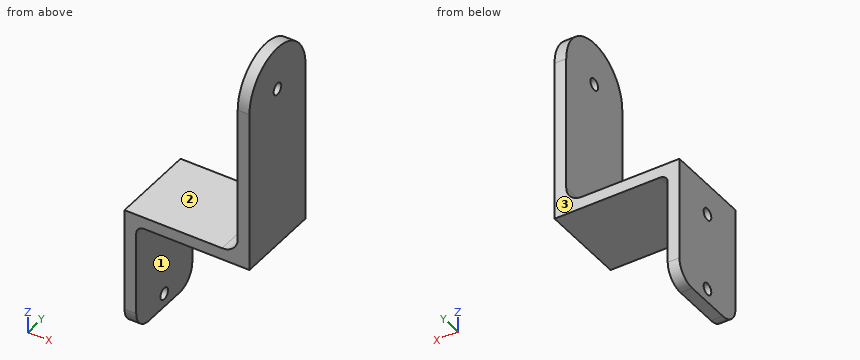
Autodesk Inventor part; units mm, degrees
ref_plane "YZ Plane" through (0, 0, 0) normal (1, 0, 0) x (0, 1, 0)
ref_plane "XZ Plane" through (0, 0, 0) normal (0, 1, 0) x (-1, 0, 0)
ref_plane "XY Plane" through (0, 0, 0) normal (0, 0, 1) x (1, 0, 0)
sketch "Sketch1" plane through (0, 0, 0) normal (1, 0, 0) x (0, 1, 0)
  circle A0 centre (0, 0) radius 1.5
  circle A1 centre (0, -20) radius 1.5
  line L0 (0, 0) -> (12, 0)
  line L1 (12, 0) -> (12, -20)
  line L2 (0, 0) -> (-12, 0)
  line L3 (-12, 0) -> (-12, -20)
  arc A2 (0, -16.5) -> (0, -23.5) centre (0, -20) ccw
  line L4 (12, -20) -> (12, -23.5)
  line L5 (12, -23.5) -> (-12, -23.5)
  line L6 (-12, -23.5) -> (-12, -20)
  line L7 (0, 0) -> (0, -1.5)
  line L8 (0, -16.5) -> (0, -20)
  line L9 (12, 0) -> (12, 5)
  line L10 (12, 5) -> (-12, 5)
  line L11 (-12, 5) -> (-12, 0)
  dimension "d0" = 3
  dimension "d1" = 20
  dimension "d2" = 3
  dimension "d3" = 12
  dimension "d4" = 12
  dimension "d5" = 7
  dimension "d6" = 5
extrude "Extrusion1" add sketch "Sketch1" along normal blind 3 contours A0 L0 L1 L4 L5 L6 L3 L2 | A0 L2 L11 L10 L9 L0
sketch "Sketch2" plane through (0, 0, 0) normal (-1, 0, 0) x (0, 0, 1)
  line L0 (-23.5, 12) -> (5, 12)
  line L1 (-23.5, -12) -> (-23.5, 12)
  line L2 (5, -12) -> (-23.5, -12)
  line L3 (5, 12) -> (5, -12)
  circle A0 centre (-20, 0) radius 1.5
  circle A1 centre (0, 0) radius 1.5
  line L4 (5, 12) -> (5, -12)
  line L5 (5, -12) -> (8, -12)
  line L6 (8, -12) -> (8, 12)
  line L7 (-23.5, 12) -> (5, 12)
  line L8 (8, 12) -> (5, 12)
  dimension "d9" = 3
extrude "Extrusion2" add sketch "Sketch2" against normal blind 32 contours L8 L6 L5 L3
sketch "Sketch3" plane through (0, -12, 8) normal (0, 0, 1) x (1, 0, 0)
  line L0 (0, 0) -> (0, 24)
  line L1 (0, 0) -> (32, 0)
  line L2 (32, 24) -> (32, 0)
  line L3 (0, 24) -> (32, 24)
  line L4 (32, 24) -> (32, 0)
  line L5 (32, 0) -> (29, 0)
  line L6 (0, 0) -> (32, 0)
  line L7 (29, 0) -> (29, 24)
  line L8 (0, 24) -> (32, 24)
  point P0 (0, 12)
  dimension "d12" = 3
extrude "Extrusion3" add sketch "Sketch3" along normal blind 50 contours L7 L3 L2 L1
sketch "Sketch4" plane through (32, 0, 0) normal (1, 0, 0) x (0, 0, -1)
  line L0 (-5, -12) -> (-5, 12)
  line L1 (-5, 12) -> (-58, 12)
  line L2 (-58, -12) -> (-58, 12)
  line L3 (-5, -12) -> (-58, -12)
  line L4 (23.5, 12) -> (-5, 12)
  line L5 (-5, 12) -> (-5, 0)
  line L6 (-5, -12) -> (-5, 12)
  line L7 (-5, 0) -> (-46.61, 0)
  circle A0 centre (-46.61, 0) radius 1.5
  point P0 (0, 0)
  dimension "d15" = 12
  dimension "d16" = 41.61
  dimension "d17" = 3
extrude "Extrusion4" cut sketch "Sketch4" against normal blind 50 contours A0
fillet "Fillet1" radius 2 1 edges at (3, 0, 5)
fillet "Fillet2" radius 4 1 edges at (29, 0, 8)
sketch "Sketch5" plane through (32, 0, 0) normal (1, 0, 0) x (0, 0, -1)
  circle A0 centre (-46.61, 0) radius 1.5
  line L0 (-5, -12) -> (-5, 12)
  line L1 (-5, 12) -> (-58, 12)
  line L2 (-58, -12) -> (-58, 12)
  line L3 (-5, -12) -> (-58, -12)
  circle A1 centre (-46.61, 0) radius 1.5
  circle A2 centre (-46.61, 0) radius 11
  line L4 (-3, 12) -> (-5, 12)
  line L5 (-5, 12) -> (-5, -12)
  line L6 (-5, -12) -> (-3, -12)
  line L7 (-3, -12) -> (-3, 12)
  line L8 (-3, -12) -> (-3, 12)
  line L9 (-3, -12) -> (23.5, -12)
  line L10 (23.5, -12) -> (23.5, 12)
  line L11 (23.5, 12) -> (-3, 12)
  circle A3 centre (20, 0) radius 1.5
  circle A4 centre (0, 0) radius 1.5
  line L12 (-46.61, 11) -> (23.5, 11)
  line L13 (23.5, -12) -> (23.5, 12)
  line L14 (-46.61, -11) -> (23.5, -11)
  dimension "d22" = 22
extrude "Extrusion5" cut sketch "Sketch5" against normal through all contours L3 L2 L1 L0 L12 A2 L14 | L0 L14 L7 L6 | L7 L14 L10 L9 | L0 L4 L7 L12 | L7 L11 L10 L12
fillet "Fillet3" radius 5 2 edges at (1.5, -11, -23.5) (1.5, 11, -23.5)
properties part number "acople_2"
Read the model definition and answer for the solid it produces. Units are mm, in the model's axes. Face numbers are marked on the shaded views. A direction names the side the tool comes from. Coordinates: 2 decimals unless noted, no trailing zeros. Write each loop counter-clockwise with the first axis right and the second up, starting at its lowest first coordinate (ties: lowest second). Pieces come first, ordered by that corner, then holes. Notation, with made-up numbers: M -7,26 L 8,26 A15 cw 8,32 Z; hole C 27.25,6.25 d11. An arc over 180 degrees is marked long. Use a Markdown table: item, result.
Q1. Which of the six approach directions +Z, -Z, +X, -X, +Y, -Y give full straight-line access (tool end or side, diameter ignored) to the marked faces 1, 2 and 3?
Answer block:
| item | result |
|---|---|
| face 1 | -Z, +X, +Y, -Y |
| face 2 | +Z, -X, +Y, -Y |
| face 3 | +Z, -Z, +X, -X, +Y |
Q2. Each of these flat-tipped pins is pushed along its axis until it touches: pin 1 Ø11 at (x, y) = (13.5, -1) entering from -Z; pin 2 Ø1 at (x, z) = (27.5, 37.5) entering from -Y; pin 3 Ø1.5 at (x, y) = (11.5, 7) entering from +Z; pin 4 Ø11 at (y, z) = (-4.5, -8) entering from +X. Where does it stop, or does it pass through?
Answer block:
| item | result |
|---|---|
| pin 1 | stops at z = 5 |
| pin 2 | passes through |
| pin 3 | stops at z = 8 |
| pin 4 | stops at x = 3 |
Q3. The part is cut by section D-D, the plane z = -20. Write down the section's boundary in (x, y).
Answer block:
| item | result |
|---|---|
| outline | M 0,-10.77 L 3,-10.77 L 3,-1.5 L 0,-1.5 Z; M 0,1.5 L 3,1.5 L 3,10.77 L 0,10.77 Z |
Q4. The part is cut by section C-C, the plane y = 7. Write down the section's boundary in (x, z), then the cut area to 3 significant figures.
Answer block:
| item | result |
|---|---|
| outline | M 0,-23.4 L 3,-23.4 L 3,3 A2 cw 5,5 L 32,5 L 32,55.1 L 29,55.1 L 29,12 A4 cw 25,8 L 0,8 Z |
| area | 327 mm2 |
Q5. Straight lines are drawn through the part: L1, parallel to Z at x = 0.8, y = 0; L2, parallel to Y at x = 1, z = 0; L3, parallel to Z at x = 24, y = 9.25. For each, find the intervals that lie inside material, in ascending order. Write a range as [from, to].
Answer block:
| item | result |
|---|---|
| L1 | z = [-23.5, -21.5], [-18.5, -1.5], [1.5, 8] |
| L2 | y = [-11, -1.5], [1.5, 11] |
| L3 | z = [5, 8] |
Q6. The part is cut by section B-B, the plane z = 0. Write down the section's boundary in (x, y), then the cut area to 3 significant figures.
Answer block:
| item | result |
|---|---|
| outline | M 0,-11 L 3,-11 L 3,-1.5 L 0,-1.5 Z; M 0,1.5 L 3,1.5 L 3,11 L 0,11 Z |
| area | 57.0 mm2 |
Q7. The part is cut by section A-A, the plane y = 0. Write down the section's boundary in (x, z).
Answer block:
| item | result |
|---|---|
| outline | M 0,-23.5 L 3,-23.5 L 3,-21.5 L 0,-21.5 Z; M 0,-18.5 L 3,-18.5 L 3,-1.5 L 0,-1.5 Z; M 0,1.5 L 3,1.5 L 3,3 A2 cw 5,5 L 32,5 L 32,45.11 L 29,45.11 L 29,12 A4 cw 25,8 L 0,8 Z; M 29,48.11 L 32,48.11 L 32,57.61 L 29,57.61 Z |
